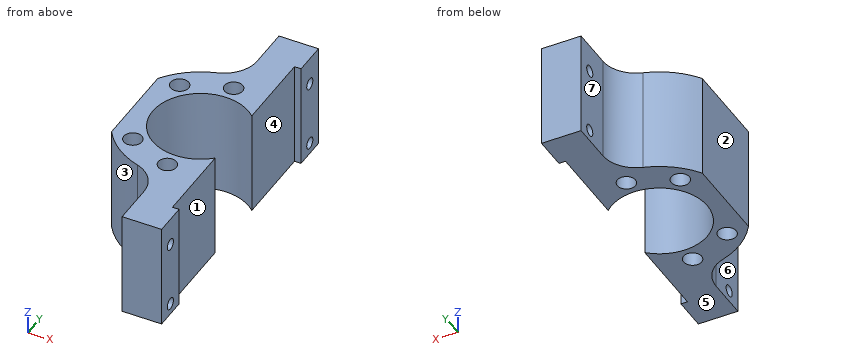
from build123d import *

# Parameters (mm, degrees)
ESQUISSE2_R        = 2.75
BOSS_EXTRU_1_DEPTH = 32
ESQUISSE3_W        = 32
ESQUISSE3_H        = 21
ESQUISSE3_R        = 1.75
BOSS_EXTRU_2_DEPTH = 10
BOSS_EXTRU_3_START = 2
ESQUISSE4_W        = 32
ESQUISSE4_H        = 10
ESQUISSE4_R        = 1.75
BOSS_EXTRU_3_DEPTH = 2
CONG_1_R           = 10


with BuildPart() as part:
    # Esquisse2 → Boss.-Extru.1 (new body)
    with BuildSketch(Plane.XY):
        with BuildLine():
            Line((-22.386521132, 12.057241029), (-22.386521132, -14.475757294))
            ThreePointArc((-22.386521132, -14.475757294), (-13.735618456, -22.356314427), (-2.386521132, -25.209258133))
            Line((-2.386521132, -25.209258133), (7.613478868, -25.209258133))
            Line((7.613478868, -25.209258133), (7.613478868, -11.709258133))
            ThreePointArc((7.613478868, -11.709258133), (-16.886521132, -1.209258133), (7.613478868, 9.290741867))
            Line((7.613478868, 9.290741867), (7.613478868, 22.790741867))
            Line((7.613478868, 22.790741867), (-2.386521132, 22.790741867))
            ThreePointArc((-2.386521132, 22.790741867), (-13.735618456, 19.937798162), (-22.386521132, 12.057241029))
        make_face()
        with Locations((-2.386521132, 17.790741867)):
            Circle(ESQUISSE2_R, mode=Mode.SUBTRACT)
        with Locations((-15.821549975, 12.22577071)):
            Circle(ESQUISSE2_R, mode=Mode.SUBTRACT)
        with Locations((-2.386521132, -20.209258133)):
            Circle(ESQUISSE2_R, mode=Mode.SUBTRACT)
        with Locations((-15.821549975, -14.644286975)):
            Circle(ESQUISSE2_R, mode=Mode.SUBTRACT)
    extrude(amount=BOSS_EXTRU_1_DEPTH)

    # Esquisse3 → Boss.-Extru.2 (add)
    # profile 1 of 2: a face of its own
    with BuildSketch(Plane(origin=(7.613478868, 0, 0), x_dir=(0, 0, -1), z_dir=(1, 0, 0))):
        with Locations((-16, 33.290741867)):
            Rectangle(ESQUISSE3_W, ESQUISSE3_H)
        with Locations(Location((-23.5, 38.790741867, 0), (0, 0, 90))):
            Circle(ESQUISSE3_R, mode=Mode.SUBTRACT)
        with Locations(Location((-3.5, 38.790741867, 0), (0, 0, 90))):
            Circle(ESQUISSE3_R, mode=Mode.SUBTRACT)
    # profile 2 of 2: a face of its own
    with BuildSketch(Plane(origin=(7.613478868, 0, 0), x_dir=(0, 0, -1), z_dir=(1, 0, 0))):
        with Locations((-16, -35.709258133)):
            Rectangle(ESQUISSE3_W, ESQUISSE3_H)
        with Locations(Location((-23.5, -41.209258133, 0), (0, 0, 90))):
            Circle(ESQUISSE3_R, mode=Mode.SUBTRACT)
        with Locations(Location((-3.5, -41.209258133, 0), (0, 0, 90))):
            Circle(ESQUISSE3_R, mode=Mode.SUBTRACT)
    extrude(amount=-BOSS_EXTRU_2_DEPTH)

    # Esquisse4 → Boss.-Extru.3 (add)
    # profile 1 of 2: a face of its own
    with BuildSketch(Plane(origin=(7.613478868, 0, 0), x_dir=(0, 0, -1), z_dir=(1, 0, 0)).offset(BOSS_EXTRU_3_START)):
        with Locations((-16, 38.790741867)):
            Rectangle(ESQUISSE4_W, ESQUISSE4_H)
        with Locations(Location((-3.5, 38.790741867, 0), (0, 0, 90))):
            Circle(ESQUISSE4_R, mode=Mode.SUBTRACT)
        with Locations(Location((-23.5, 38.790741867, 0), (0, 0, 90))):
            Circle(ESQUISSE4_R, mode=Mode.SUBTRACT)
    # profile 2 of 2: a face of its own
    with BuildSketch(Plane(origin=(7.613478868, 0, 0), x_dir=(0, 0, -1), z_dir=(1, 0, 0)).offset(BOSS_EXTRU_3_START)):
        with Locations((-16, -41.209258133)):
            Rectangle(ESQUISSE4_W, ESQUISSE4_H)
        with Locations(Location((-3.5, -41.209258133, 0), (0, 0, 90))):
            Circle(ESQUISSE4_R, mode=Mode.SUBTRACT)
        with Locations(Location((-23.5, -41.209258133, 0), (0, 0, 90))):
            Circle(ESQUISSE4_R, mode=Mode.SUBTRACT)
    extrude(amount=-BOSS_EXTRU_3_DEPTH)

    # Congé1
    cong_1_edges = [part.edges().sort_by_distance(p)[0] for p in [
        (-2.386521132, 22.790741867, 16),
        (-2.386521132, -25.209258133, 16),
    ]]
    fillet(cong_1_edges, radius=CONG_1_R)


solid = part.part
Design review of the part built by this model. Coordinates are the model's own, in mm. Face numbers are marked on the shaded views. A direction names the side the tool comes from. Coordinates: 2 decimals unless noted, no trailing zeros. Loops run counter-clockwise (first coordinate to the right, second up) from the corner with the lowest first, then second, coordinate; pieces in that order, holes last. Notation, with made-up numbers: (3, -9) -> (36, -9) arc R14 cw to (36, 10) -> close; hole circle Ø1 at (-4, 6). An arc over 180 degrees is marked (long way). Use a Markdown table: item, result. Add a question column.
Item 1: We need section D-D, the plane z = 10.5. Write out the cut boundary in (x, y).
Item 2: We need section B-B, the plane x = -6. Write out the cut boundary in (y, z), and give its area (3 significant figures).
Item 3: We need section A-A, the plane z = 23.5. Write out the cut boundary in (x, y), and give its area (3 significant figures).
Item 4: Clearance check with flat-ended pins moving along their axes: P1, Ø10, axis at y = -41.5, z = 9, coming from the -X side; P2, Ø3, axis at y = 38.79, z = 23.5, coming from the +X side; P3, Ø4, axis at y = 22, z = 14, coming from the -X side; P4, Ø12, axis at y = -18, z = 23.5, coming from the +X side. State where each tip first meets the part, or that it passes through.
Item 5: The part is to be moulded in two halves that separate along Y. For the marked faces 1, 2, 3 and 4, say which applies: +Y half, -Y half, draft (parallel to the pull), parting line (faces both ways), or undercut.
Item 6: Wall thickness on L1, parallel to Y at x = -17.5, z = 16; L2, parallel to X at y = 39, z = 6.5; L3, parallel to X at y = 31.5, z = 28: over which ranges is each line inside the solid? List them lowest first. Write a range as from..to.
Item 7: Machinability: for the marked faces 5, 6 and 7, which of the approach directions +Z, -Z, +X, -X, +Y, -Y give a long, thin tool a straight path to every point of the face, cutting with its end or side? Answer none if there is none.
Item 8: We need section C-C, the plane x = -12. Write out the cut boundary in (y, z), and give its area (3 significant figures).
Numbers:
| question | item | result |
|---|---|---|
| 1 | outline | (-22.39, -14.48) arc R24 ccw to (-9.45, -24.15) arc R10 cw to (-2.39, -33.71) -> (-2.39, -46.21) -> (9.61, -46.21) -> (9.61, -36.21) -> (7.61, -36.21) -> (7.61, -11.71) arc R14.5 cw (long way) to (7.61, 9.29) -> (7.61, 33.79) -> (9.61, 33.79) -> (9.61, 43.79) -> (-2.39, 43.79) -> (-2.39, 31.29) arc R10 cw to (-9.45, 21.73) arc R24 ccw to (-22.39, 12.06) -> close; hole circle Ø5.5 at (-15.82, -14.64); hole circle Ø5.5 at (-15.82, 12.23); hole circle Ø5.5 at (-2.39, -20.21); hole circle Ø5.5 at (-2.39, 17.79) |
| 2 | outline | (-26.01, 0) -> (-15.25, 0) -> (-15.25, 32) -> (-26.01, 32) -> close; (12.83, 0) -> (23.59, 0) -> (23.59, 32) -> (12.83, 32) -> close |
| 2 | area | 689 mm^2 |
| 3 | outline | (-22.39, -14.48) arc R24 ccw to (-9.45, -24.15) arc R10 cw to (-2.39, -33.71) -> (-2.39, -39.46) -> (9.61, -39.46) -> (9.61, -36.21) -> (7.61, -36.21) -> (7.61, -11.71) arc R14.5 cw (long way) to (7.61, 9.29) -> (7.61, 33.79) -> (9.61, 33.79) -> (9.61, 37.04) -> (-2.39, 37.04) -> (-2.39, 31.29) arc R10 cw to (-9.45, 21.73) arc R24 ccw to (-22.39, 12.06) -> close; (-2.39, -46.21) -> (9.61, -46.21) -> (9.61, -42.96) -> (-2.39, -42.96) -> close; (-2.39, 40.54) -> (9.61, 40.54) -> (9.61, 43.79) -> (-2.39, 43.79) -> close; hole circle Ø5.5 at (-15.82, -14.64); hole circle Ø5.5 at (-15.82, 12.23); hole circle Ø5.5 at (-2.39, -20.21); hole circle Ø5.5 at (-2.39, 17.79) |
| 3 | area | 1,020 mm^2 |
| 4 | P1 | stops at x = -2.39 |
| 4 | P2 | passes through |
| 4 | P3 | stops at x = -13.62 |
| 4 | P4 | stops at x = 7.61 |
| 5 | face 1 | undercut |
| 5 | face 2 | draft |
| 5 | face 3 | -Y half |
| 5 | face 4 | undercut |
| 6 | L1 | y = -19.85..-16.82, -12.47..10.05, 14.4..17.43 |
| 6 | L2 | x = -2.39..9.61 |
| 6 | L3 | x = -2.39..7.61 |
| 7 | face 5 | -Z, +X, -X, +Y, -Y |
| 7 | face 6 | +Z, -Z, -X, -Y |
| 7 | face 7 | +Z, -Z, -X, +Y |
| 8 | outline | (-23.2, 0) -> (-12.06, 0) -> (-12.06, 32) -> (-23.2, 32) -> close; (9.65, 0) -> (20.78, 0) -> (20.78, 32) -> (9.65, 32) -> close |
| 8 | area | 713 mm^2 |
